Build history of the part. All positions in model axes, mm. A direction names the side the tool comes from. Coordinates: 2 decimals unless noted, no trailing zeros. Order: outer loops, then holes, each group sorted by start corner. A loop starts at its lowest first (then second) coordinate and runs counter-clockwise, first axis right, second up. Notation, with made-up numbers: (-25, 32) - (5, 32) arc R9 ccw to (5, 37) - close; hole circle Ø4 at (17, 39.25). An arc over 180 degrees is marked (long way). One line per item, written item: value.
Autodesk Inventor part; units mm, degrees
ref_plane "YZ Plane" through (0, 0, 0) normal (1, 0, 0) x (0, 1, 0)
ref_plane "XZ Plane" through (0, 0, 0) normal (0, 1, 0) x (-1, 0, 0)
ref_plane "XY Plane" through (0, 0, 0) normal (0, 0, 1) x (1, 0, 0)
sketch "Sketch1" plane through (0, 0, 0) normal (0, 0, 1) x (1, 0, 0)
  line L0 (24.1218, -9.7086) -> (-26.6782, -9.7086)
  line L1 (-26.6782, -9.7086) -> (-26.6782, 15.6914)
  line L2 (-26.6782, 15.6914) -> (24.1218, 15.6914)
  line L3 (24.1218, 15.6914) -> (24.1218, -9.7086)
  line L4 (21.5818, 13.1514) -> (-24.1382, 13.1514)
  line L5 (-24.1382, 13.1514) -> (-24.1382, -7.1686)
  line L6 (-24.1382, -7.1686) -> (21.5818, -7.1686)
  line L7 (21.5818, -7.1686) -> (21.5818, 13.1514)
  point P0 (0, 0)
  dimension "d0" = 25.4
  dimension "d1" = 50.8
  dimension "d2" = 2.54
extrude "Extrusion1" add sketch "Sketch1" along normal blind 762
sketch "Sketch2" plane through (24.1218, -9.7086, 0) normal (1, 0, 0) x (0, 0, -1)
  circle A0 centre (-12.7, 12.7) radius 2.0701
  line L0 (0, 25.4) -> (-762, 25.4)
  line L1 (0, 25.4) -> (0, 0)
  circle A1 centre (-38.1, 12.7) radius 2.0701
  circle A2 centre (-63.5, 12.7) radius 2.0701
  circle A3 centre (-88.9, 12.7) radius 2.0701
  circle A4 centre (-114.3, 12.7) radius 2.0701
  circle A5 centre (-139.7, 12.7) radius 2.0701
  circle A6 centre (-165.1, 12.7) radius 2.0701
  circle A7 centre (-190.5, 12.7) radius 2.0701
  circle A8 centre (-215.9, 12.7) radius 2.0701
  circle A9 centre (-241.3, 12.7) radius 2.0701
  circle A10 centre (-266.7, 12.7) radius 2.0701
  circle A11 centre (-292.1, 12.7) radius 2.0701
  circle A12 centre (-317.5, 12.7) radius 2.0701
  circle A13 centre (-342.9, 12.7) radius 2.0701
  circle A14 centre (-368.3, 12.7) radius 2.0701
  circle A15 centre (-393.7, 12.7) radius 2.0701
  circle A16 centre (-419.1, 12.7) radius 2.0701
  circle A17 centre (-444.5, 12.7) radius 2.0701
  circle A18 centre (-469.9, 12.7) radius 2.0701
  circle A19 centre (-495.3, 12.7) radius 2.0701
  circle A20 centre (-520.7, 12.7) radius 2.0701
  circle A21 centre (-546.1, 12.7) radius 2.0701
  circle A22 centre (-571.5, 12.7) radius 2.0701
  circle A23 centre (-596.9, 12.7) radius 2.0701
  circle A24 centre (-622.3, 12.7) radius 2.0701
  circle A25 centre (-647.7, 12.7) radius 2.0701
  circle A26 centre (-673.1, 12.7) radius 2.0701
  circle A27 centre (-698.5, 12.7) radius 2.0701
  circle A28 centre (-723.9, 12.7) radius 2.0701
  circle A29 centre (-749.3, 12.7) radius 2.0701
  point P0 (0, 9.7086)
  point P1 (0, 12.7)
  dimension "d5" = 12.7
  dimension "d6" = 4.1402
  dimension "d9" = 25.4
extrude "Extrusion2" cut sketch "Sketch2" against normal through all
sketch "Sketch3" plane through (-26.6782, -9.7086, 0) normal (0, -1, 0) x (1, 0, 0)
  circle A0 centre (25.4, 736.6) radius 9.525
  circle A1 centre (25.4, 535.9) radius 9.525
  line L0 (0, 762) -> (50.8, 762)
  point P0 (26.6782, 0)
  point P1 (25.4, 762)
  dimension "d16" = 19.05
  dimension "d17" = 200.7
  dimension "d18" = 25.4
extrude "Extrusion3" cut sketch "Sketch3" against normal through all
properties part number "30inVersaFrameUpright"
1. 3-axis set-ups, long thin cutter, end or side, ignore diameter. For faces 4 (the face through (-2, -7.169, 376)), 5 (the face through (-8.299, 14.404, 743.037)): which of +Z, -Z, +X, -X, +Y, -Y reach the whole face in a straight line?
Values found:
face 4: +Z, -Z
face 5: +Y, -Y
2. Band-saw the part on A-A, the plane y = -3. Give the cut face in (x, z).
Values found:
outline: (-26.68, 0) - (-24.14, 0) - (-24.14, 762) - (-26.68, 762) - close; (21.58, 0) - (24.12, 0) - (24.12, 762) - (21.58, 762) - close
3. Flat gauge pins, fed straight in: P1, Ø12, axis at x = -3, z = 544.5, coming from the -Y side; P2, Ø3.5, axis at y = 2.99, z = 444.5, coming from the -X side. Where does each tip first touch, or does it go through?
Values found:
P1: stops at y = -9.71
P2: passes through
4. Band-saw the part on B-B, the plane z = 461. Give the cut face in (x, y).
Values found:
outline: (-26.68, -9.71) - (24.12, -9.71) - (24.12, 15.69) - (-26.68, 15.69) - close; hole (-24.14, -7.17) - (21.58, -7.17) - (21.58, 13.15) - (-24.14, 13.15) - close
5. Two-plate mould, pull along Z, no slides. Class faces 1 (the face through (-1.4, 13.4, 0)), 2 (the face through (-3.34, -8.46, 526.6)), 3 (the face through (-2, 15.691, 376)): pulls with the +Z half, pulls with the -Z half, needs draft (parallel to the pull), parting line crosses it, or undercut.
Values found:
face 1: pulls with the -Z half
face 2: undercut
face 3: needs draft
6. Band-saw the part on C-C, the plane x = 1. Give the cut face in (y, z).
Values found:
outline: (-9.71, 0) - (-7.17, 0) - (-7.17, 526.65) - (-9.71, 526.65) - close; (-9.71, 545.15) - (-7.17, 545.15) - (-7.17, 727.35) - (-9.71, 727.35) - close; (-9.71, 745.85) - (-7.17, 745.85) - (-7.17, 762) - (-9.71, 762) - close; (13.15, 0) - (15.69, 0) - (15.69, 526.65) - (13.15, 526.65) - close; (13.15, 545.15) - (15.69, 545.15) - (15.69, 727.35) - (13.15, 727.35) - close; (13.15, 745.85) - (15.69, 745.85) - (15.69, 762) - (13.15, 762) - close
7. Probe line 1 along X through (y, z) = (3.5, 103); line 2 along Y through (x, z) = (-8, 403); line 3 along X through (y, z) = (14.5, 535.9). List the from-to ranges inside material, lowest first.
Values found:
line 1: x = -26.68 to -24.14, 21.58 to 24.12
line 2: y = -9.71 to -7.17, 13.15 to 15.69
line 3: x = -26.68 to -10.8, 8.25 to 24.12
